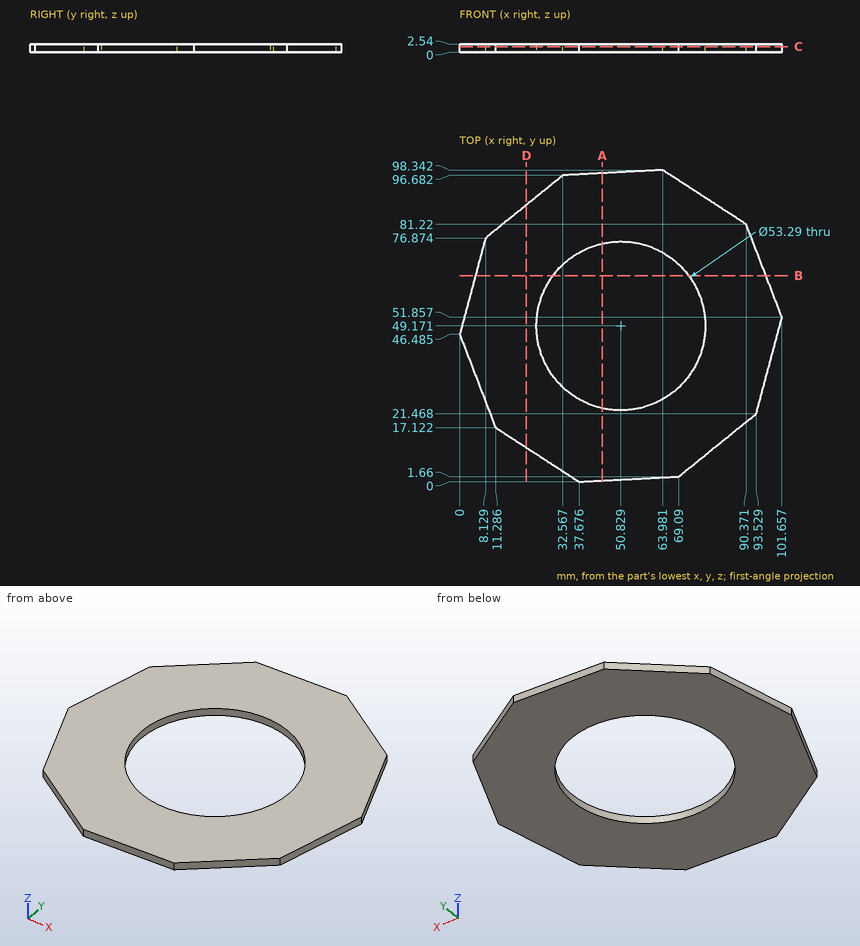
The figure shows three views and two pictorial views of one solid part (mm, origin at its lowest corner). Answer the questions. Coordinates: 2 decimals unless noted, no trailing zeros. Order: outer loops, then holes, each group sorted by start corner. A loop starts at its lowest first (then second) coordinate and runs counter-clockwise, first axis right, second up.
Q1. A cutting plane is placed at C-C, the plane z = 1.75. Write down the section's boundary in (x, y) (1 decimal), and give its area (3 significant figures).
Q2. A cutting plane is placed at D-D, the plane x = 21. Write down the section's boundary in (y, z).
Q3. Consider line 1 (Y direction, x = 57, z = 0.2); line 2 (X direction, y = 51, z = 2.45) (1 decimal); line 3 (X direction, y = 64.5, z = 2.3) (1 decimal). Determine where each line is inside the solid, lowest interval first.
Q4. A cutting plane is placed at B-B, the plane y = 65. Write down the section's boundary in (x, z) (1 decimal), and give its area (3 significant figures).
Q5. A cutting plane is placed at A-A, the plane x = 45. Write down the section's boundary in (y, z), and give its area (3 significant figures).
Q6. Given P1, Ø1.5, axis at x = 61, z = 0.5, coming from the -Y side; P2, Ø1.5, axis at x = 46, z = 1.5, coming from the +Y side, each flat-ended and moving along its own axis, determine where each tip first touches the part or whether it passes through.
Answers follow:
1. outline: (0, 46.5) - (11.3, 17.1) - (37.7, 0) - (69.1, 1.7) - (93.5, 21.5) - (101.7, 51.9) - (90.4, 81.2) - (64, 98.3) - (32.6, 96.7) - (8.1, 76.9) - close; hole circle Ø53.3 at (50.8, 49.2)
1. area: 5,380 mm2
2. outline: (10.82, 0) - (87.31, 0) - (87.31, 2.54) - (10.82, 2.54) - close
3. line 1: y = 1.02 to 23.25, 75.09 to 97.97
3. line 2: x = 1.2 to 24.2, 77.4 to 101.4
3. line 3: x = 4.8 to 29, 72.6 to 96.8
4. outline: (5, 0) - (29.4, 0) - (29.4, 2.5) - (5, 2.5) - close; (72.3, 0) - (96.6, 0) - (96.6, 2.5) - (72.3, 2.5) - close
4. area: 124 mm2
5. outline: (0.39, 0) - (23.17, 0) - (23.17, 2.54) - (0.39, 2.54) - close; (75.17, 0) - (97.34, 0) - (97.34, 2.54) - (75.17, 2.54) - close
5. area: 114 mm2
6. P1: stops at y = 1.19
6. P2: stops at y = 97.43
